Geometry: final body of the model. Coordinates: model frame, mm. A direction names the side the tool comes from. Give positions to 0.01 mm unless a question says otherwise; leave off trailing zeros. Answer in a Markdown table with one row per item. Add a question column.
Q1. Line query: line 1 along Z through (x, y) = (0.1, 6.5); line 2 along Z through (x, y) = (0.25, 10.5); line 3 along Z through (x, y) = (0.65, 5.75). Output: solid intervals per line, ascending. Write a range as from..to.
Q2. Cut plane A-A on y = 8.75. Count the separate pieces of the cut face and the enclosed holes in it, and give its area (3 significant figures).
Q3. Contact query for flat-ended pins moving along their axis: P1, Ø3, axis at y = -2.5, z = 23, coming from the +X side; P2, Ø1.5, axis at x = 1, y = 4, coming from the -Z side. Output: stop coordinate, or through.
Q4. Set-up query: faces 1 (the face through (0, 4, 31)), 2 (the face through (1.25, 13.36, 32.97)). Return all of +Z, -Z, +X, -X, +Y, -Y with unobstructed straight access to the full face (end or side cutting, diameter ignored); none if empty.
from build123d import *

# Parameters (mm, degrees)
F1_DEPTH = 2.54


with BuildPart() as f1:
    # F0 (on Right) → F1 (new body)
    with BuildSketch(Plane.YZ):
        with BuildLine():
            add(Edge.make_bspline(
                [(4.3062982129, 18.4064569529), (4.4145754331, 17.851669978), (4.5227315225, 17.2993939442), (4.6310087426, 16.7446069692)],
                knots=[0, 0, 0, 0, 1.6932756114, 1.6932756114, 1.6932756114, 1.6932756114], degree=3))
            add(Edge.make_bspline(
                [(4.1593257549, 19.1126760485), (4.2081809899, 18.7562347142), (4.274320241, 18.4384364203), (4.3062982129, 18.4064569529)],
                knots=[0, 0, 0, 0, 1, 1, 1, 1], degree=3))
            add(Edge.make_bspline(
                [(4.587080479, 20.5390156251), (4.1199305204, 19.8352235894), (4.0789979985, 19.6987369871), (4.1593257549, 19.1126760485)],
                knots=[0, 0, 0, 0, 1, 1, 1, 1], degree=3))
            add(Edge.make_bspline(
                [(5.5515264837, 21.5446767853), (5.3052015891, 21.4196091783), (4.8712005131, 20.9670619552), (4.587080479, 20.5390156251)],
                knots=[0, 0, 0, 0, 1, 1, 1, 1], degree=3))
            add(Edge.make_bspline(
                [(6.1705583504, 21.9085323912), (6.0764144472, 21.8334789664), (5.7978513782, 21.6697458878), (5.5515264837, 21.5446767853)],
                knots=[0, 0, 0, 0, 1, 1, 1, 1], degree=3))
            add(Edge.make_bspline(
                [(7.6551638138, 22.5023530426), (6.9327747869, 22.2508031651), (6.2647022536, 21.9835843206), (6.1705583504, 21.9085323912)],
                knots=[0, 0, 0, 0, 1, 1, 1, 1], degree=3))
            add(Edge.make_bspline(
                [(12.8379490604, 25.3474205293), (11.0188744075, 24.1153788353), (8.8182758107, 22.907369969), (7.6551638138, 22.5023530426)],
                knots=[0, 0, 0, 0, 1, 1, 1, 1], degree=3))
            add(Edge.make_bspline(
                [(14.1645862732, 26.7650134187), (13.7263112988, 26.182685038), (13.1293263476, 25.5447690602), (12.8379490604, 25.3474205293)],
                knots=[0, 0, 0, 0, 1, 1, 1, 1], degree=3))
            add(Edge.make_bspline(
                [(15.0707260149, 28.8437191762), (14.9687566007, 27.8920215914), (14.9081429111, 27.7529688556), (14.1645862732, 26.7650134187)],
                knots=[0, 0, 0, 0, 1, 1, 1, 1], degree=3))
            add(Edge.make_bspline(
                [(13.7717031507, 32.4500579966), (14.9154480174, 30.9995061424), (15.2131509134, 30.1730242108), (15.0707260149, 28.8437191762)],
                knots=[0, 0, 0, 0, 1, 1, 1, 1], degree=3))
            Line((13.7717031507, 32.4500579966), (12.9332459293, 33.5134287489))
            add(Edge.make_bspline(
                [(5.7822467141, 36.1096769875), (6.3762820613, 35.8425612862), (7.6581101579, 35.2661706512), (10.0985801685, 33.9916505274), (11.9792064067, 33.6743798154), (12.9332459293, 33.5134287489)],
                knots=[0, 0, 0, 0, 0.2985104209, 0.6441351452, 1, 1, 1, 1], degree=3))
            add(Edge.make_bspline(
                [(2.3612512264, 38.0030753022), (3.524023764, 37.060348717), (3.9435058477, 36.828180924), (5.7822467141, 36.1096769875)],
                knots=[0, 0, 0, 0, 1, 1, 1, 1], degree=3))
            add(Edge.make_bspline(
                [(0.8822565632, 40.104596619), (0.8822565632, 39.355544328), (1.1336105412, 38.9983941666), (2.3612512264, 38.0030753022)],
                knots=[0, 0, 0, 0, 1, 1, 1, 1], degree=3))
            add(Edge.make_bspline(
                [(1.8150057341, 42.0706138216), (1.1379322929, 41.3211757133), (0.8822565632, 40.7822712173), (0.8822565632, 40.104596619)],
                knots=[0, 0, 0, 0, 1, 1, 1, 1], degree=3))
            add(Edge.make_bspline(
                [(5.130764324, 43.3401306362), (3.05388746, 43.1938311152), (2.7112413368, 43.0626412758), (1.8150057341, 42.0706138216)],
                knots=[0, 0, 0, 0, 1, 1, 1, 1], degree=3))
            add(Edge.make_bspline(
                [(8.0668398269, 43.2044874484), (7.1214319611, 43.4407407174), (6.7817796603, 43.4564321157), (5.130764324, 43.3401306362)],
                knots=[0, 0, 0, 0, 1, 1, 1, 1], degree=3))
            add(Edge.make_bspline(
                [(10.7201501424, 41.0876351286), (10.9152779809, 41.9986469351), (10.0136334591, 42.7179927908), (8.0668398269, 43.2044874484)],
                knots=[0, 0, 0, 0, 1, 1, 1, 1], degree=3))
            add(Edge.make_bspline(
                [(9.665690573, 40.3289329193), (10.5618693499, 40.5852172833), (10.6217697262, 40.6283181582), (10.7201501424, 41.0876351286)],
                knots=[0, 0, 0, 0, 1, 1, 1, 1], degree=3))
            add(Edge.make_bspline(
                [(7.5720919693, 40.2786809659), (8.6570311041, 40.0685451343), (8.7641507304, 40.0711157541), (9.665690573, 40.3289329193)],
                knots=[0, 0, 0, 0, 1, 1, 1, 1], degree=3))
            add(Edge.make_bspline(
                [(6.0726310451, 39.9564846541), (5.8181157581, 40.4320493175), (6.2742280524, 40.5300558798), (7.5720919693, 40.2786809659)],
                knots=[0, 0, 0, 0, 1, 1, 1, 1], degree=3))
            add(Edge.make_bspline(
                [(6.5300473421, 39.4837029595), (6.3592693595, 39.5927561585), (6.153431353, 39.8055074725), (6.0726310451, 39.9564846541)],
                knots=[0, 0, 0, 0, 1, 1, 1, 1], degree=3))
            add(Edge.make_bspline(
                [(10.1351419765, 38.422938717), (8.9017319771, 38.5991465544), (7.0723090467, 39.1374364346), (6.5300473421, 39.4837029595)],
                knots=[0, 0, 0, 0, 1, 1, 1, 1], degree=3))
            add(Edge.make_bspline(
                [(12.5184609466, 38.5560277345), (11.4262137148, 38.2780015199), (11.2273892084, 38.2668980574), (10.1351419765, 38.422938717)],
                knots=[0, 0, 0, 0, 1, 1, 1, 1], degree=3))
            add(Edge.make_bspline(
                [(15.8478038939, 40.1600989773), (15.3262417352, 39.4728148369), (14.4370196327, 39.0443901666), (12.5184609466, 38.5560277345)],
                knots=[0, 0, 0, 0, 1, 1, 1, 1], degree=3))
            add(Edge.make_bspline(
                [(16.1916538269, 42.665268915), (16.5742081122, 41.8004400355), (16.459741508, 40.9664720523), (15.8478038939, 40.1600989773)],
                knots=[0, 0, 0, 0, 1, 1, 1, 1], degree=3))
            add(Edge.make_bspline(
                [(9.3640681921, 45.169465337), (13.687454414, 44.6991854732), (15.6026887907, 43.9967228622), (16.1916538269, 42.665268915)],
                knots=[0, 0, 0, 0, 1, 1, 1, 1], degree=3))
            add(Edge.make_bspline(
                [(0.6018660961, 44.4634840126), (3.9265493277, 45.1443049658), (7.1831702034, 45.4066951126), (9.3640681921, 45.169465337)],
                knots=[0, 0, 0, 0, 1, 1, 1, 1], degree=3))
            add(Edge.make_bspline(
                [(-6.869657556, 41.234824422), (-5.2947947751, 42.7188122786), (-2.9319959009, 43.7398283685), (0.6018660961, 44.4634840126)],
                knots=[0, 0, 0, 0, 1, 1, 1, 1], degree=3))
            add(Edge.make_bspline(
                [(-8.5345189474, 39.0052730794), (-8.3623113473, 39.6899925817), (-8.0137224416, 40.156818035), (-6.869657556, 41.234824422)],
                knots=[0, 0, 0, 0, 1, 1, 1, 1], degree=3))
            add(Edge.make_bspline(
                [(-8.7753407118, 36.4924825027), (-8.8935279106, 36.8100804109), (-8.7745930039, 38.0504859655), (-8.5345189474, 39.0052730794)],
                knots=[0, 0, 0, 0, 1, 1, 1, 1], degree=3))
            add(Edge.make_bspline(
                [(-8.7281162361, 36.3415613512), (-8.7359523782, 36.3815132341), (-8.7524901075, 36.4310764124), (-8.7753407118, 36.4924825027)],
                knots=[0.7856250085, 0.7856250085, 0.7856250085, 0.7856250085, 1, 1, 1, 1], degree=3))
            add(Edge.make_bspline(
                [(-8.7281162361, 36.3415613512), (-8.6458521412, 36.079976454), (-8.4223909985, 35.3950724639), (-7.7740737011, 33.9365337451), (-7.1033373756, 33.4345247336), (-6.8248215993, 33.2504152378)],
                knots=[0.0477039482, 0.0477039482, 0.0477039482, 0.0477039482, 0.2946798893, 0.6733320976, 0.9307398592, 0.9307398592, 0.9307398592, 0.9307398592], degree=3))
            add(Edge.make_bspline(
                [(-6.5989783193, 33.1045596313), (-6.6784388414, 33.1576214869), (-6.7534797046, 33.2061446456), (-6.8248215993, 33.2504152378)],
                knots=[0, 0, 0, 0, 0.1293994473, 0.1293994473, 0.1293994473, 0.1293994473], degree=3))
            add(Edge.make_bspline(
                [(-1.7070350009, 31.5580125491), (-4.1254349308, 31.8328086656), (-5.2061584884, 32.1744708052), (-6.5989783193, 33.1045596313)],
                knots=[0, 0, 0, 0, 1, 1, 1, 1], degree=3))
            add(Edge.make_bspline(
                [(-0.0876372414, 31.2203327018), (-0.3512072712, 31.3347993061), (-1.0799368612, 31.4867544896), (-1.7070350009, 31.5580125491)],
                knots=[0, 0, 0, 0, 1, 1, 1, 1], degree=3))
            add(Edge.make_bspline(
                [(1.2231171599, 30.6940734419), (0.7657711475, 30.8690505521), (0.1759312931, 31.1058660975), (-0.0876372414, 31.2203327018)],
                knots=[0, 0, 0, 0, 1, 1, 1, 1], degree=3))
            add(Edge.make_bspline(
                [(3.0494864513, 28.81478288), (2.9324193189, 29.7517625823), (2.4863203289, 30.2107879467), (1.2231171599, 30.6940734419)],
                knots=[0, 0, 0, 0, 1, 1, 1, 1], degree=3))
            add(Edge.make_bspline(
                [(2.3150428774, 26.1949070715), (3.0131418651, 27.3668106181), (3.1634206875, 27.9028798057), (3.0494864513, 28.81478288)],
                knots=[0, 0, 0, 0, 1, 1, 1, 1], degree=3))
            add(Edge.make_bspline(
                [(1.1052768976, 24.8880422468), (1.5894491744, 25.2096807685), (1.9785115095, 25.6299688814), (2.3150428774, 26.1949070715)],
                knots=[0, 0, 0, 0, 1, 1, 1, 1], degree=3))
            add(Edge.make_bspline(
                [(-2.2063049959, 21.2954821878), (-1.9664672152, 22.606247057), (-1.3928810353, 23.228498554), (1.1052768976, 24.8880422468)],
                knots=[0, 0, 0, 0, 1, 1, 1, 1], degree=3))
            add(Edge.make_bspline(
                [(-2.1212277989, 19.9286152985), (-2.3103276161, 20.4012205339), (-2.3254582334, 20.6443003762), (-2.2063049959, 21.2954821878)],
                knots=[0, 0, 0, 0, 1, 1, 1, 1], degree=3))
            add(Edge.make_bspline(
                [(-2.29458986, 18.2876431748), (-1.924623985, 18.8522822818), (-1.8757343555, 19.3150626353), (-2.1212277989, 19.9286152985)],
                knots=[0, 0, 0, 0, 1, 1, 1, 1], degree=3))
            add(Edge.make_bspline(
                [(-2.29458986, 18.2876431748), (-2.29458986, 17.7030911022), (-2.29458986, 17.1185390296), (-2.29458986, 16.533986957)],
                knots=[0, 0, 0, 0, 1.7536562178, 1.7536562178, 1.7536562178, 1.7536562178], degree=3))
            add(Edge.make_bspline(
                [(-0.0965289838, 16.5494406097), (-0.8129556754, 16.5571901602), (-1.5605586109, 16.551185881), (-2.29458986, 16.533986957)],
                knots=[0, 0, 0, 0, 0.2456952601, 0.2456952601, 0.2456952601, 0.2456952601], degree=3))
            add(Edge.make_bspline(
                [(3.8289375551, 16.681698176), (3.0978347403, 16.5935120095), (1.3313747977, 16.5339959551), (-0.0965289838, 16.5494406097)],
                knots=[0, 0, 0, 0, 1, 1, 1, 1], degree=3))
            add(Edge.make_bspline(
                [(4.6310087426, 16.7446069692), (4.3124459161, 16.729239125), (4.0494007129, 16.7082907732), (3.8289375551, 16.681698176)],
                knots=[0.7704771185, 0.7704771185, 0.7704771185, 0.7704771185, 1, 1, 1, 1], degree=3))
        make_face()
    extrude(amount=F1_DEPTH)


solid = f1.part
Completed:
| question | item | result |
|---|---|---|
| 1 | line 1 | z = 22.07..35.79, 39.5..40.41, 43.41..45.23 |
| 1 | line 2 | z = 23.89..34.02, 38.37..40.64, 42..45.03 |
| 1 | line 3 | z = 21.65..36.12, 43.38..45.19 |
| 2 | separate pieces | 3 |
| 2 | enclosed holes | 0 |
| 2 | area | 39.1 mm² |
| 3 | P1 | stops at x = 2.54 |
| 3 | P2 | stops at z = 16.63 |
| 4 | face 1 | +Z, -Z, -X, +Y, -Y |
| 4 | face 2 | +X, -X, +Y |
